For this review, take the finished solid that the model builds, in its own axes (mm). A direction names the side the tool comes from. Give positions to 0.01 mm unless a question says otherwise; leave off trailing zeros. Order: outer loops, then holes, each group sorted by start corner. A loop starts at its lowest first (then second) coordinate and runs counter-clockwise, first axis right, second up. Notation, with made-up numbers: (10, 75) - (61, 75) arc R18 cw to (61, 101) - close; hole circle Ø10 at (76.25, 49). An arc over 180 degrees is marked (long way). One line per item, written item: value.
```python
from build123d import *

# Parameters (mm, degrees)
BOSS_EXTRUDE1_DEPTH = 5
SKETCH3_W           = 8
SKETCH3_H           = 4
BOSS_EXTRUDE2_DEPTH = 3
FILLET1_START       = -3.841593316
FILLET1_DEPTH       = 8
CUT_EXTRUDE1_START  = -10
CUT_EXTRUDE1_DEPTH  = 10


with BuildPart() as part:
    # Sketch1 → Boss-Extrude1 (new body)
    with BuildSketch(Plane(origin=(0, 0, 0), x_dir=(1, 0, 0), z_dir=(0, 1, 0))):
        with BuildLine():
            Line((-30, 0), (30, 0))
            ThreePointArc((30, 0), (0, 30), (-30, 0))
        make_face()
    extrude(amount=BOSS_EXTRUDE1_DEPTH)

    # Sketch3 → Boss-Extrude2 (add)
    with BuildSketch(Plane(origin=(0, 5, 0), x_dir=(1, 0, 0), z_dir=(0, 1, 0))):
        with Locations((0.158406684, 24.731666579)):
            Rectangle(SKETCH3_W, SKETCH3_H)
    extrude(amount=BOSS_EXTRUDE2_DEPTH)

    # Fillet1: read off the stored shape, not the designer's step
    # Fillet1 outline → Fillet1 (cut)
    with BuildSketch(Plane.YZ.offset(FILLET1_START)):
        with BuildLine():
            Line((8, -22.731666579), (5, -22.731666579))
            add(Edge.make_bspline(
                [(5, -22.731666579), (8, -23.506263249), (8, -26.604649926)],
                knots=[0, 0, 0, 1, 1, 1], degree=2, weights=[1, 0.057495957, 1]))
            Line((8, -26.604649926), (8, -22.731666579))
        make_face()
    extrude(amount=FILLET1_DEPTH, mode=Mode.SUBTRACT)

    # Sketch5 → Cut-Extrude1 (cut)
    with BuildSketch(Plane(origin=(0, 5, 0), x_dir=(1, 0, 0), z_dir=(0, 1, 0)).offset(CUT_EXTRUDE1_START)):
        with BuildLine():
            Line((-21.393876913, 0), (-21.393876913, 6))
            Line((-21.393876913, 6), (-29.393876913, 6))
            ThreePointArc((-29.393876913, 6), (-29.84808459, 3.01526886), (-30, 0))
            Line((-30, 0), (-21.393876913, 0))
        make_face()
        with BuildLine():
            Line((21.393876913, 6), (29.393876913, 6))
            ThreePointArc((29.393876913, 6), (29.84808459, 3.01526886), (30, 0))
            Line((30, 0), (21.393876913, 0))
            Line((21.393876913, 0), (21.393876913, 6))
        make_face()
    extrude(amount=CUT_EXTRUDE1_DEPTH, mode=Mode.SUBTRACT)


solid = part.part
```
(1) Take a section at A-A (y = 2.75). Write out the cut boundary in (x, z).
Answers below:
outline: (-29.39, -6) arc R30 ccw to (29.39, -6) - (21.39, -6) - (21.39, 0) - (-21.39, 0) - (-21.39, -6) - close
(2) Wall thickness on line 1 (Y direction, x = -22, z = -18); line 2 (Z direction, x = -6, y = 2); line 3 (Z direction, x = -24, y = 1): over which ranges is each line inside the solid? List them lowest first. Write a range as from..to.
Answers below:
line 1: y = 0..5
line 2: z = -29.39..0
line 3: z = -18..-6
(3) Take a section at C-C (x = -13.5). Write out the cut boundary in (y, z), then the cut area to 3 significant figures.
Answers below:
outline: (0, -26.79) - (5, -26.79) - (5, 0) - (0, 0) - close
area: 134 mm^2
(4) Take a section at B-B (z = -20). Write out the cut boundary in (x, y).
Answers below:
outline: (-22.36, 0) - (22.36, 0) - (22.36, 5) - (-22.36, 5) - close
(5) For P1, Ø1, axis at x = -22.5, z = -12.5, coming from the +Y side; P2, Ø1.5, axis at y = 7, z = -24, coming from the -X side; P3, Ø2.5, axis at y = 2, z = -4, coming from the +X side, all flat-tipped, find the tip position at first contact; note any pin that passes through.
Answers below:
P1: stops at y = 5
P2: stops at x = -3.84
P3: stops at x = 21.39
(6) Machinability: for faces 1 (the face through (0, 6, -26.732)), 2 (the face through (25, 2, -6)), 3 (the face through (-25, 2, -6)), which of the approach directions +Z, -Z, +X, -X, +Y, -Y give a long, thin tool a straight path to every point of the face, cutting with its end or side? Answer none if there is none.
Answers below:
face 1: -Z, +X, -X, +Y
face 2: +Z, +X, +Y, -Y
face 3: +Z, -X, +Y, -Y
